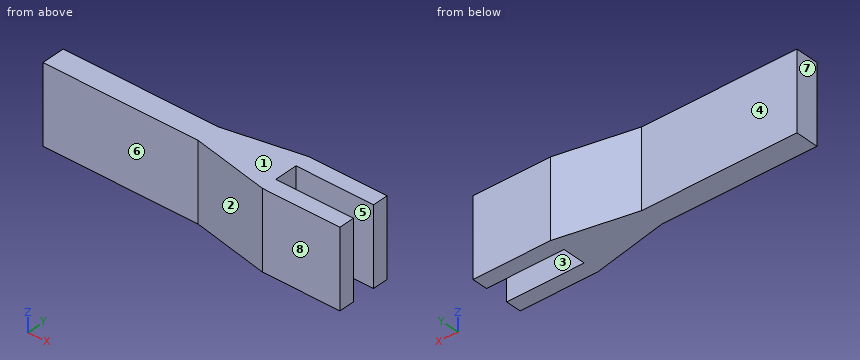
Autodesk Inventor part; units mm, degrees
ref_plane "YZ Plane" through (0, 0, 0) normal (1, 0, 0) x (0, 1, 0)
ref_plane "XZ Plane" through (0, 0, 0) normal (0, 1, 0) x (-1, 0, 0)
ref_plane "XY Plane" through (0, 0, 0) normal (0, 0, 1) x (1, 0, 0)
sketch "Sketch1" plane through (0, 0, 0) normal (0, 1, 0) x (-1, 0, 0)
  line L0 (0, 0) -> (30, 0)
  line L1 (30, 0) -> (30, 10)
  line L2 (30, 10) -> (0, 10)
  line L3 (0, 10) -> (0, 0)
  dimension "d0" = 30
  dimension "d1" = 10
extrude "Extrusion1" add sketch "Sketch1" along normal blind 3
sketch "Sketch2" plane through (0, 3, 0) normal (0, 1, 0) x (1, 0, 0)
  line L0 (-30, -10) -> (0, -10)
  line L1 (-10, -10) -> (10, -10)
  line L2 (10, -10) -> (10, 0)
  line L3 (10, 0) -> (-10, 0)
  line L4 (-10, 0) -> (-10, -10)
  line L5 (0, -10) -> (0, 0)
  dimension "d4" = 10
  dimension "d5" = 10
  dimension "d6" = 20
extrude "Extrusion2" add sketch "Sketch2" along normal blind 2
sketch "Sketch3" plane through (0, 0, 0) normal (0, -1, 0) x (1, 0, 0)
  line L0 (-10, 10) -> (10, 10)
  line L1 (10, 0) -> (0, 0)
  line L2 (-10, 10) -> (10, 10)
  line L3 (10, 10) -> (10, 0)
  line L4 (10, 0) -> (-10, 0)
  line L5 (-10, 0) -> (-10, 10)
extrude "Extrusion3" add sketch "Sketch3" along normal blind 2
sketch "Sketch4" plane through (-30, 0, 10) normal (0, 0, 1) x (1, 0, 0)
  line L0 (20, 0) -> (20, -2)
  line L1 (20, 0) -> (30, -2)
  line L2 (40, -2) -> (20, -2)
  line L3 (0, 3) -> (20, 3)
  line L4 (20, 3) -> (30, 5)
  line L5 (20, 5) -> (40, 5)
  line L6 (30, 3) -> (30, 5)
  line L7 (30, 3) -> (20, 3)
  line L8 (30, 0) -> (30, 3)
  line L9 (30, -2) -> (30, 0)
  line L10 (30, 0) -> (20, 0)
  line L11 (20, 3) -> (20, 5)
  line L12 (20, 3) -> (20, 5)
  line L13 (20, 5) -> (30, 5)
  line L14 (30, -2) -> (20, -2)
  line L15 (20, -2) -> (20, 0)
extrude "Extrusion4" cut sketch "Sketch4" against normal through all contours L1 L2 L0 | L4 L11 L5
properties part number "MotorHållare"
Geometry check sheet. Reference: the model listing, model coordinates, mm. Face numbers are marked on the shaded views. A direction names the side the tool comes from. Round coordinates to 2 decimals unless told otherwise and drop trailing zeros. Loops run counter-clockwise (first coordinate to the right, second up) from the corner with the lowest first, then second, coordinate; pieces in that order, holes last.
Item 1: Cross-section at C-C on x = -15. Record the boundary of the cut face in (y, z), then the cut area to 3 significant figures.
Item 2: Cross-section at A-A on z = 3. Record the boundary of the cut face in (x, y), then the cut area to 3 significant figures.
Item 3: Gauge pin test, flat ends, axial feed: pin 1 (4 mm diameter, centred on x = -8.5, z = 6.5, fed in from -Y); pin 2 (5 mm diameter, centred on x = -20.5, z = 4.5, fed in from -Y); pin 3 (4 mm diameter, centred on x = -7, z = 2.5, fed in from -Y). Record the tip position at first contact, or that the pin passes through.
Item 4: Access from +Z, -Z, +X, -X, +Y, -Y to the whole of each face (thin tool, end or side, straight path). Record for the marked faces 4, 5, 6, 7 and 8.
Item 5: Thickness scan on line 1 (Y direction, x = 4, z = 9.75); line 2 (X direction, y = 0.75, z = 2); line 3 (Y direction, x = -25.5, z = 5.25). Record the ranges inside material, lowest first.
Item 6: Mould release check, pull along Y, two halves, no side actions. Record for the marked faces 1, 2 and 3: pulls with the +Y half, pulls with the -Y half, needs draft (parallel to the pull), parting line crosses it, or undercut.
Item 7: Cross-section at B-B on y = -0.5. Record the boundary of the cut face in (x, z).
Answer sheet:
1. outline: (0, 0) - (3, 0) - (3, 10) - (0, 10) - close
1. area: 30.0 mm2
2. outline: (-30, 0) - (-10, 0) - (0, -2) - (10, -2) - (10, 0) - (0, 0) - (0, 3) - (10, 3) - (10, 5) - (0, 5) - (-10, 3) - (-30, 3) - close
2. area: 150 mm2
3. pin 1: stops at y = -0.7
3. pin 2: stops at y = 0
3. pin 3: stops at y = -1
4. face 4: +Z, -Z, -X, +Y
4. face 5: +Z, -Z, +X
4. face 6: +Z, -Z, -X, -Y
4. face 7: +Z, -Z, -X, +Y, -Y
4. face 8: +Z, -Z, +X, -X, -Y
5. line 1: y = -2 to 0, 3 to 5
5. line 2: x = -30 to 0
5. line 3: y = 0 to 3
6. face 1: needs draft
6. face 2: pulls with the -Y half
6. face 3: undercut
7. outline: (-7.5, 0) - (10, 0) - (10, 10) - (-7.5, 10) - close
